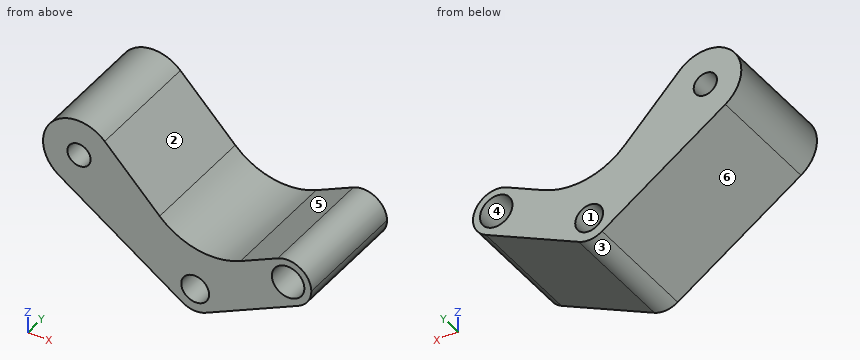
```python
from build123d import *

# Parameters (mm, degrees)
F0_R     = 5
F0_R_2   = 6
F0_R_3   = 7
F1_DEPTH = 25


with BuildPart() as f1:
    # F0 (on Front) → F1 (new body, symmetric)
    with BuildSketch(Plane.XZ):
        with BuildLine():
            ThreePointArc((-38.937303, 50.856645), (-61.936842, 49.887456), (-58.607353, 27.109559))
            ThreePointArc((-58.607353, 27.109559), (-42.691237, 26.33135), (-34.5, 40))
            ThreePointArc((-34.5, 40), (-35.652147, 45.864222), (-38.937303, 50.856645))
        make_face()
        with Locations((-50, 40)):
            Circle(F0_R, mode=Mode.SUBTRACT)
        with BuildLine():
            ThreePointArc((-5.553131, -8.316414), (-4.715331, 8.818484), (10, 0))
            ThreePointArc((10, 0), (8.506508, -5.257311), (4.472136, -8.944272))
            Line((4.472136, -8.944272), (44.472136, 11.055728))
            ThreePointArc((44.472136, 11.055728), (31.055728, 15.527864), (35.527864, 28.944272))
            Line((35.527864, 28.944272), (19.532285, 20.946482))
            ThreePointArc((19.532285, 20.946482), (1.171282, 18.189588), (-15.295793, 26.766436))
            Line((-15.295793, 26.766436), (-38.937303, 50.856645))
            ThreePointArc((-38.937303, 50.856645), (-35.652147, 45.864222), (-34.5, 40))
            ThreePointArc((-34.5, 40), (-42.691237, 26.33135), (-58.607353, 27.109559))
            Line((-58.607353, 27.109559), (-5.553131, -8.316414))
        make_face()
        with BuildLine():
            ThreePointArc((4.472136, -8.944272), (8.506508, -5.257311), (10, 0))
            ThreePointArc((10, 0), (-4.715331, 8.818484), (-5.553131, -8.316414))
            ThreePointArc((-5.553131, -8.316414), (-0.625051, -9.980446), (4.472136, -8.944272))
        make_face()
        Circle(F0_R_2, mode=Mode.SUBTRACT)
        with BuildLine():
            ThreePointArc((35.527864, 28.944272), (31.055728, 15.527864), (44.472136, 11.055728))
            ThreePointArc((44.472136, 11.055728), (48.506508, 14.742689), (50, 20))
            ThreePointArc((50, 20), (45.257311, 28.506508), (35.527864, 28.944272))
        make_face()
        with Locations((40, 20)):
            Circle(F0_R_3, mode=Mode.SUBTRACT)
    extrude(amount=F1_DEPTH, both=True)


solid = f1.part
```
Could you check a few things on this model? Use its own coordinates, in mm. Face numbers are marked on the shaded views. A direction names the side the tool comes from. Round coordinates to 2 decimals unless told otherwise and drop trailing zeros. Order: outer loops, then holes, each group sorted by start corner. A loop starts at its lowest first (then second) coordinate and runs counter-clockwise, first axis right, second up. Notation, with made-up numbers: (12.5, -39.75) -> (70.5, -39.75) arc R26 cw to (70.5, -7.75) -> close; hole circle Ø5 at (13.5, 82.25). An arc over 180 degrees is marked (long way). One line per question, with ' | ' between items.
Q1. If we section it at B-B on x = -50: Write out the boundary of the cut face in (y, z).
Computed values:
outline: (-25, 21.36) -> (25, 21.36) -> (25, 35) -> (-25, 35) -> close; (-25, 45) -> (25, 45) -> (25, 55.5) -> (-25, 55.5) -> close
Q2. If I drill on line 1 (X direction, y = -10, z = 2); line 2 (X direction, y = 15.5, z = 1.5); line 3 (Z direction, x = 0, y = 3), over which ranges is the centre line in solid material (lowest first)? Write a range as from..to.
Computed values:
line 1: -21..-5.66, 5.66..26.36 | line 2: -20.25..-5.81, 5.81..25.36 | line 3: -10..-6, 6..18.41
Q3. If we section it at A-A on y = 5.5: Write out the boundary of the cut face in (x, z).
Computed values:
outline: (-58.61, 27.11) -> (-5.55, -8.32) arc R10 ccw to (4.47, -8.94) -> (44.47, 11.06) arc R10 ccw to (35.53, 28.94) -> (19.53, 20.95) arc R30 cw to (-15.3, 26.77) -> (-38.94, 50.86) arc R15.5 ccw (long way) to start; hole circle Ø10 at (-50, 40); hole circle Ø12 at (0, 0); hole circle Ø14 at (40, 20)
Q4. I'm going to push flat-ended pins straight in: pin 1 (1.5 mm diameter, centred on x = 31.5, z = 1.5, fed in from -Y); pin 2 (4 mm diameter, centred on y = -6.5, z = 33.5, fed in from +X); pin 3 (2 mm diameter, centred on y = 5.5, z = 25.5, fed in from +X); pin 4 (6 mm diameter, centred on x = -16, y = -1.5, fed in from -Z). Where does each tip first touch, or does it pass through?
Computed values:
pin 1: through | pin 2: x = -19.94 | pin 3: x = 48.93 | pin 4: z = -3.34
Q5. If we section it at D-D on z = 25: Write out the boundary of the cut face in (x, y), plus the area to 3 significant figures.
Computed values:
outline: (-55.45, -25) -> (-13.41, -25) -> (-13.41, 25) -> (-55.45, 25) -> close; (27.64, -25) -> (35.1, -25) -> (35.1, 25) -> (27.64, 25) -> close; (44.9, -25) -> (48.66, -25) -> (48.66, 25) -> (44.9, 25) -> close | area: 2,660 mm²
Q6. We'd pull the mould along Z, two halves only. Please class the marked faces 1, 2, 3 and 4: released by +Z, released by -Z, zero draft, split by the parting line, or undercut.
Computed values:
face 1: undercut | face 2: released by +Z | face 3: released by -Z | face 4: undercut
Q7. If we section it at C-C on z = 40: Write out the boundary of the cut face in (x, y).
Computed values:
outline: (-65.5, -25) -> (-55, -25) -> (-55, 25) -> (-65.5, 25) -> close; (-45, -25) -> (-28.28, -25) -> (-28.28, 25) -> (-45, 25) -> close
Q8. Which directions (+Z, -Z, +X, -X, +Y, -Y) give clear straight access to the entire face, cutting with the end or side of a thin tool? Please do the marked faces 5 and 6.
Computed values:
face 5: +Z, +Y, -Y | face 6: -Z, -X, +Y, -Y
